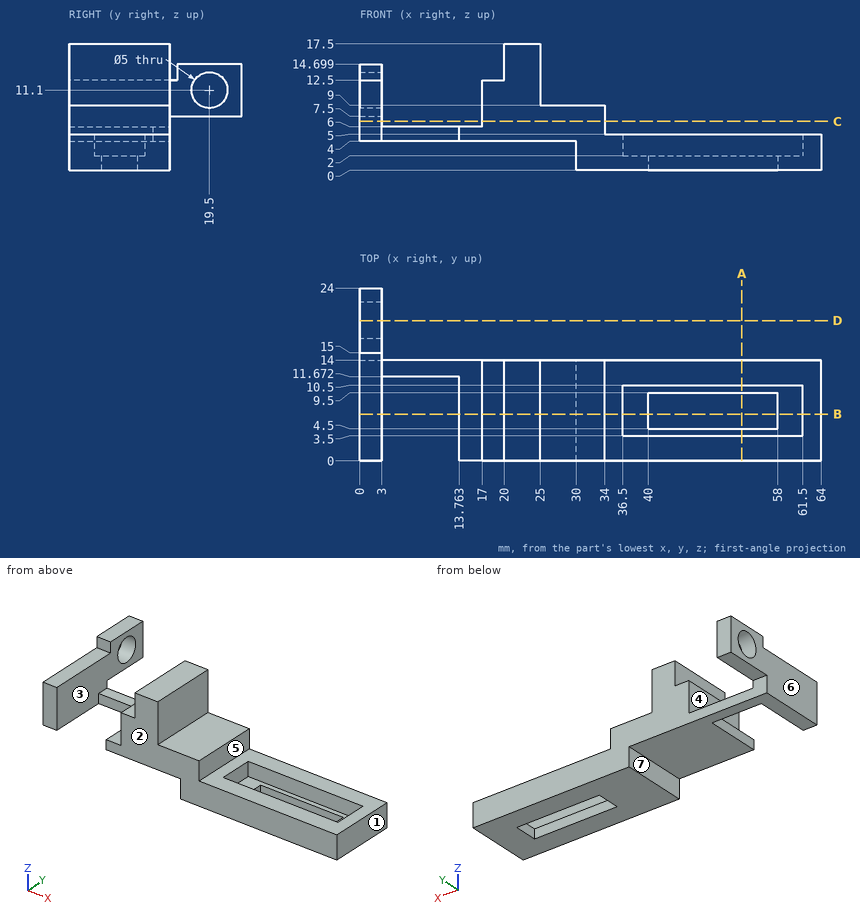
Input: dimensioned drawing with shaded views. Units: mm. Origin: part minimum x, y, z. A direction names the side the tool comes from. Give positions to 0.01 mm unless a question says otherwise; leave off trailing zeros. Order: outer loops, then holes, each group sorted by start corner. A loop starts at its lowest first (then second) coordinate and runs counter-clockwise, first axis right, second up. Notation, with made-up numbers: (-31.75, 85.5) -> (23.25, 85.5) arc R19 cw to (23.25, 96.5) -> close; hole circle Ø5 at (59, 18.5). An arc over 180 degrees is marked (long way). Write item = value, one per line.
Item 1: Section query B-B (y = 6.5). Output: boundary loops of the cut face in (x, z).
Check result:
outline = (0, 4) -> (3, 4) -> (3, 12.5) -> (0, 12.5) -> close; (13.76, 4) -> (30, 4) -> (30, 0) -> (40, 0) -> (40, 2) -> (36.5, 2) -> (36.5, 5) -> (34, 5) -> (34, 9) -> (25, 9) -> (25, 17.5) -> (20, 17.5) -> (20, 12.5) -> (17, 12.5) -> (17, 6) -> (13.76, 6) -> close; (58, 0) -> (64, 0) -> (64, 5) -> (61.5, 5) -> (61.5, 2) -> (58, 2) -> close
Item 2: Set-up query: the marked faces 4, 5, 6 and 7. Return all of +Z, -Z, +X, -X, +Y, -Y with unobstructed straight access to the full face (end or side cutting, diameter ignored); none if empty.
Check result:
face_4 = +Z, +Y, -Y
face_5 = +Z, +X, +Y, -Y
face_6 = +Z, -Z, -X, +Y, -Y
face_7 = -Z, -X, +Y, -Y
Item 3: Section query C-C (z = 6.75). Output: boundary loops of the cut face in (x, y).
Check result:
outline = (0, 0) -> (3, 0) -> (3, 14) -> (0, 14) -> close; (17, 0) -> (34, 0) -> (34, 14) -> (17, 14) -> close
Item 4: Section query D-D (y = 19.5). Output: boundary loops of the cut face in (x, z).
Check result:
outline = (0, 7.5) -> (3, 7.5) -> (3, 8.6) -> (0, 8.6) -> close; (0, 13.6) -> (3, 13.6) -> (3, 14.7) -> (0, 14.7) -> close
Item 5: Section query A-A (x = 53). Output: boundary loops of the cut face in (y, z), then the cut area to 3 significant figures.
Check result:
outline = (0, 0) -> (4.5, 0) -> (4.5, 2) -> (3.5, 2) -> (3.5, 5) -> (0, 5) -> close; (9.5, 0) -> (14, 0) -> (14, 5) -> (10.5, 5) -> (10.5, 2) -> (9.5, 2) -> close
area = 39.0 mm²
Item 6: Contact query for flat-ended pins moving along their axis: pin 1 (8 mm diameter, centred on x = 24, y = 7.5, fed in from -Z); pin 2 (1.5 mm diameter, centred on y = 8.5, z = 15, fed in from -X); pin 3 (1 mm diameter, centred on x = 52, z = 1, fed in from +Y); pin 4 (10 mm diameter, centred on x = 44, y = 21, fed in from -Z). Output: stop coordinate, or through.
Check result:
pin_1 = 4
pin_2 = 20
pin_3 = 14
pin_4 = through
Item 7: Mould query, pull axis X, two halves, no side actions, for the marked faces 1, 2 and 3. Classes: +X half, -X half, draft (parallel to the pull), parting line (faces both ways), or undercut.
Check result:
face_1 = +X half
face_2 = draft
face_3 = undercut
Item 8: Ray query, probe 1 along X at (y, z) = (9.5, 10.5); probe 2 along Y at (x, z) = (58.5, 2.5); probe 3 along X at (y, z) = (6.75, 7.75). Return the intervals inside material, ascending.
Check result:
probe_1 = 0 to 3, 17 to 25
probe_2 = 0 to 3.5, 10.5 to 14
probe_3 = 0 to 3, 17 to 34
